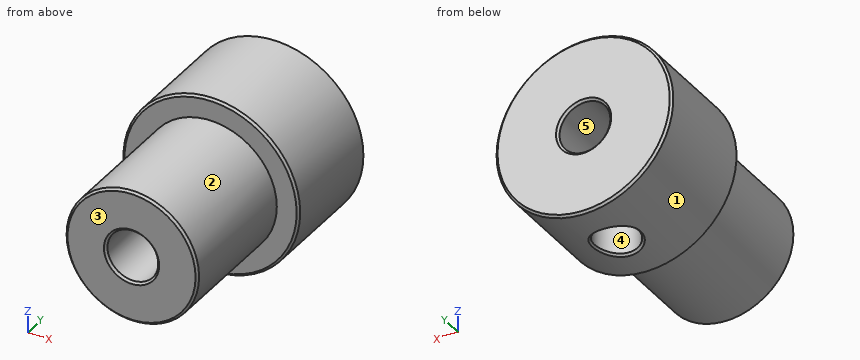
Autodesk Inventor part; units mm, degrees
ref_plane "YZ Plane" through (0, 0, 0) normal (1, 0, 0) x (0, 1, 0)
ref_plane "XZ Plane" through (0, 0, 0) normal (0, 1, 0) x (-1, 0, 0)
ref_plane "XY Plane" through (0, 0, 0) normal (0, 0, 1) x (1, 0, 0)
sketch "Skizze1" plane through (0, 0, 0) normal (0, 0, 1) x (1, 0, 0)
  line L0 (0, 5) -> (4, 5)
  line L1 (4, 5) -> (4, 0)
  line L2 (4, 0) -> (3, 0)
  line L3 (3, 0) -> (3, -6)
  line L4 (3, -6) -> (0, -6)
  line L5 (0, -6) -> (0, 5)
  point P0 (0, 0)
  dimension "d0" = 6
  dimension "d1" = 6
  dimension "d2" = 8
  dimension "d3" = 5
revolve "Umdrehung1" add sketch "Skizze1" angle 360 about axis through (0, -6, 0) along (0, 1, 0)
chamfer "Fase1" distance 0.1 angle 45 3 edges at (-4, 5, 0) (-3, -6, 0) (-4, 0, 0)
hole "Bohrung1" at (0, 5, 0) direction (0, -1, 0) diameter 2.3 end through all both
chamfer "Fase2" distance 0.1 angle 45 2 edges at (0, -6, -1.15) (0, 5, -1.15)
sketch "Skizze2" plane through (0, 0, 0) normal (0, 0, 1) x (1, 0, 0)
  circle A0 centre (0, 2.5) radius 1
  line L0 (1.25, 5) -> (-1.25, 5)
  line L1 (0, 7.2) -> (0, -8.2)
  point P0 (0, 0)
  dimension "d20" = 2
  dimension "d21" = 2.5
extrude "Extrusion1" cut sketch "Skizze2" against normal blind 10
chamfer "Fase3" distance 0.1 angle 45 1 edges at (-1, 2.5012, -3.873)
thread "Gewinde1"
properties part number "nabe" material "Aluminium 6061"
Design review of the part built by this model. Coordinates are the model's own, in mm. Face numbers are marked on the shaded views. A direction names the side the tool comes from. Round coordinates to 2 decimals unless told otherwise and drop trailing zeros. Loops run counter-clockwise (first coordinate to the right, second up) from the corner with the lowest first, then second, coordinate; pieces in that order, holes last. Notation, with made-up numbers: (-3.75, -29) -> (30.25, -29) arc R25 cw to (30.25, 4) -> close; hole circle Ø4 at (78.5, 36.25). An arc over 180 degrees is marked (long way). Use one line per item in the form item = value. Start each with the question number.
Q1. Wall thickness on line 1 along X through (y, z) = (-2.25, 0); line 2 along Y through (x, z) = (0, -1.45): over which ranges is each line inside the solid? List them lowest first. Write a range as [from, to].
Q2. We need section C-C on x = 0. State how many separate pieces and enclosed holes the cut face has, then the cut area to 3 significant figures.
Q3. We need section B-B on y = -2. Give the boundary of the cut face in (x, z).
Q4. We need section D-D on y = 3.75. Give the boundary of the cut face in (x, z), then the cut area to 3 significant figures.
Q5. Draft analysis for pull direction Y (two halves, no side actions). For the marked faces 3, 4 and 5, state which applies: +Y half, -Y half, draft (parallel to the pull), parting line (faces both ways), or undercut.
Q6. Machinability: for the marked faces 1 and 2, which of the approach directions +Z, -Z, +X, -X, +Y, -Y give a long, thin tool a straight path to every point of the face, cutting with its end or side? Answer none if there is none.
Q7. We need section A-A on z = 0. Give the boundary of the cut face in (x, y).
Q8. For pin 1 Ø1.5 at (y, z) = (0.5, 2) entering from -X; pin 2 Ø1.4 at (x, z) = (0, 0) entering from +Y, all flat-tipped, find the tip position at first contact; note any pin that passes through.
Calculated:
q1.line_1 = [-3, -1.15], [1.15, 3]
q1.line_2 = [-6, 1.5], [3.5, 5]
q2.separate_pieces = 3
q2.enclosed_holes = 0
q2.area = 44.9 mm²
q3.outline = circle Ø6 at (0, 0); hole circle Ø2.3 at (0, 0)
q4.outline = circle Ø8 at (0, 0); hole circle Ø2.3 at (0, 0)
q4.area = 46.1 mm²
q5.face_3 = -Y half
q5.face_4 = undercut
q5.face_5 = draft
q6.face_1 = +Y, -Y
q6.face_2 = -Y
q7.outline = (-4, 0.1) -> (-3.9, 0) -> (-3, 0) -> (-3, -5.9) -> (-2.9, -6) -> (-1.25, -6) -> (-1.15, -5.9) -> (-1.15, 4.9) -> (-1.25, 5) -> (-3.9, 5) -> (-4, 4.9) -> close; (1.15, -5.9) -> (1.25, -6) -> (2.9, -6) -> (3, -5.9) -> (3, 0) -> (3.9, 0) -> (4, 0.1) -> (4, 4.9) -> (3.9, 5) -> (1.25, 5) -> (1.15, 4.9) -> close
q8.pin_1 = -3.8
q8.pin_2 = through
